from build123d import *

# Parameters (mm, degrees)
F0_W      = 101.6
F0_H      = 63.5
F1_DEPTH  = 12.7
F2_R      = 5.08
F3_W      = 101.6
F3_H      = 25.4
F4_DEPTH  = 63.5
F5_W      = 25.4
F5_H      = 25.4
F6_DEPTH  = 38.1
F8_DEPTH  = 25.4
F9_W      = 50.8
F9_H      = 25.4
F10_DEPTH = 50.8
F12_DEPTH = 25.4
F14_DEPTH = 50.8
F15_R     = 12.7
F16_DEPTH = 25.4
F17_R     = 6.35
F18_DEPTH = 25.4


with BuildPart() as f1:
    # F0 (on Top) → F1 (new body)
    with BuildSketch(Plane.XY):
        with Locations((8.665344, 7.042157)):
            Rectangle(F0_W, F0_H)
    extrude(amount=F1_DEPTH)

    # F2
    f2_edges = [f1.edges().sort_by_distance(p)[0] for p in [
        (59.465344, -24.707843, 6.35),
        (-42.134656, -24.707843, 6.35),
    ]]
    fillet(f2_edges, radius=F2_R)

    # F3 (on face) → F4 (join)
    with BuildSketch(Plane.XY.offset(12.7)):
        with Locations((8.665344, 26.092157)):
            Rectangle(F3_W, F3_H)
    extrude(amount=F4_DEPTH)

    # F5 (on face) → F6 (cut)
    with BuildSketch(Plane.XY.offset(76.2)):
        with Locations((-29.434656, 26.092157)):
            Rectangle(F5_W, F5_H)
        with Locations((46.765344, 26.092157)):
            Rectangle(F5_W, F5_H)
    extrude(amount=-F6_DEPTH, mode=Mode.SUBTRACT)

    # F7 (on face) → F8 (cut)
    with BuildSketch(Plane.XZ.offset(-13.392157)):
        with BuildLine():
            Line((-42.134656, 38.1), (-42.134656, 12.7))
            ThreePointArc((-42.134656, 12.7), (-24.174144, 20.139488), (-16.734656, 38.1))
            Line((-16.734656, 38.1), (-42.134656, 38.1))
        make_face()
        with BuildLine():
            Line((59.465344, 38.1), (34.065344, 38.1))
            ThreePointArc((34.065344, 38.1), (41.504832, 20.139488), (59.465344, 12.7))
            Line((59.465344, 12.7), (59.465344, 38.1))
        make_face()
    extrude(amount=-F8_DEPTH, mode=Mode.SUBTRACT)

    # F9 (on face) → F10 (join)
    with BuildSketch(Plane.XY.offset(76.2)):
        with Locations((8.665344, 0.692157)):
            Rectangle(F9_W, F9_H)
        with Locations((8.665344, 26.092157)):
            Rectangle(F9_W, F9_H)
    extrude(amount=F10_DEPTH)

    # F11 (on face) → F12 (cut)
    with BuildSketch(Plane.XZ.offset(12.007843)):
        with BuildLine():
            Line((-16.734656, 76.2), (8.665344, 76.2))
            ThreePointArc((8.665344, 76.2), (-9.295168, 83.639488), (-16.734656, 101.6))
            Line((-16.734656, 101.6), (-16.734656, 76.2))
        make_face()
        with BuildLine():
            Line((34.065344, 76.2), (34.065344, 101.6))
            ThreePointArc((34.065344, 101.6), (26.625856, 83.639488), (8.665344, 76.2))
            Line((8.665344, 76.2), (34.065344, 76.2))
        make_face()
    extrude(amount=-F12_DEPTH, mode=Mode.SUBTRACT)

    # F13 (on face) → F14 (cut)
    with BuildSketch(Plane.XZ.offset(12.007843)):
        with BuildLine():
            ThreePointArc((-16.734656, 101.6), (-9.295168, 119.560512), (8.665344, 127))
            Line((8.665344, 127), (-16.734656, 127))
            Line((-16.734656, 127), (-16.734656, 101.6))
        make_face()
        with BuildLine():
            ThreePointArc((8.665344, 127), (26.625856, 119.560512), (34.065344, 101.6))
            Line((34.065344, 101.6), (34.065344, 127))
            Line((34.065344, 127), (8.665344, 127))
        make_face()
    extrude(amount=-F14_DEPTH, mode=Mode.SUBTRACT)

    # F15 (on face) → F16 (cut)
    with BuildSketch(Plane.XZ.offset(12.007843)):
        with Locations((8.665344, 101.6)):
            Circle(F15_R)
    extrude(amount=-F16_DEPTH, mode=Mode.SUBTRACT)

    # F17 (on face) → F18 (cut)
    with BuildSketch(Plane.XY.offset(12.7)):
        with Locations((-29.434656, -12.007843)):
            Circle(F17_R)
        with Locations((46.765344, -12.007843)):
            Circle(F17_R)
    extrude(amount=-F18_DEPTH, mode=Mode.SUBTRACT)


solid = f1.part
Can you work these out from the model? Positions are in its coordinate system, mm. A direction names the side the tool comes from. Give positions to 0.01 mm unless a question says otherwise; leave off trailing zeros. Order: outer loops, then holes, each group sorted by start corner. A loop starts at its lowest first (then second) coordinate and runs counter-clockwise, first axis right, second up. Notation, with made-up numbers: M 64,-26.5 L 121,-26.5 A19 ccw 121,-0.5 Z; hole C -10.5,-26.5 d6. An arc over 180 degrees is marked long. One line per question, with ' | ' between items.
Item 1: We'd pull the mould along X, two halves only. Please class faces 4 (the face through (-16.735, 26, 69)), 5 (the face through (7.01, 0.51, 114.19)), 6 (the face through (34.065, 26, 69)): released by +X, released by -X, zero draft, split by the parting line, or undercut.
Answer block:
face 4: released by -X | face 5: undercut | face 6: released by +X
Item 2: I'm going to push flat-ended pins straight in: pin 1 Ø4 at (x, y) = (0.5, 31) entering from -Z; pin 2 Ø6 at (x, z) = (20, 55) entering from -Y; pin 3 Ø12.5 at (y, z) = (29.5, 74) entering from -X; pin 4 Ø5 at (x, y) = (-1.5, -13) entering from +Z. Where does each tip first touch, or does it pass through?
Answer block:
pin 1: stops at z = 0 | pin 2: stops at y = 13.39 | pin 3: stops at x = -16.73 | pin 4: stops at z = 125.75
Item 3: Suppose I cut it at A-A, the plane y = 27. Write out the boundary of the cut face in (x, z), then the cut area to 3 significant figures.
Answer block:
outline: M -42.13,0 L 59.47,0 L 59.47,12.7 A25.4 cw 34.07,38.1 L 34.07,101.6 A25.4 ccw 8.67,127 A25.4 ccw -16.73,101.6 L -16.73,38.1 A25.4 cw -42.13,12.7 Z | area: 7,100 mm2
Item 4: Suppose I cut it at B-B, the plane x = -24.5. Write out the boundary of the cut face in (y, z).
Answer block:
outline: M -24.71,0 L -16,0 L -16,12.7 L -24.71,12.7 Z; M -8.01,0 L 38.79,0 L 38.79,19.82 L 13.39,19.82 L 13.39,12.7 L -8.01,12.7 Z
Item 5: For faces 1 (the face through (-3, -12.008, 107)), 2 (the face through (8, 13.392, 102)), 3 (the face through (8, -5, 12.7)), which set-ups out of +Z, -Z, +X, -X, +Y, -Y let a thin tool reach every point of the face, with its end or its side?
Answer block:
face 1: +Z, +X, -X, -Y | face 2: -Y | face 3: +X, -X, -Y
Item 6: Please list where these lines run through material, in increasing order: L1, parallel to Z at x = 17.5, y = -2; L2, parallel to X at y = 20, z = 99.5; L3, parallel to Z at x = 40, y = -15.
Answer block:
L1: z = 0 to 12.7, 77.79 to 92.48, 110.72 to 125.41 | L2: x = -16.73 to 34.07 | L3: z = 0 to 12.7
Item 7: Suppose I cut it at D-D, the plane x = 26.5. Write out the boundary of the cut face in (y, z), then the cut area to 3 significant figures.
Answer block:
outline: M -24.71,0 L 38.79,0 L 38.79,119.69 L -12.01,119.69 L -12.01,83.51 L 13.39,83.51 L 13.39,12.7 L -24.71,12.7 Z | area: 4,440 mm2
Item 8: Suppose I cut it at C-C, the plane z = 51.5. Write out the boundary of the cut face in (x, y).
Answer block:
outline: M -16.73,13.39 L 34.07,13.39 L 34.07,38.79 L -16.73,38.79 Z
